from build123d import *

# Parameters (mm, degrees)
SKETCH1_R           = 278.5
BOSS_EXTRUDE1_DEPTH = 2.25
FILLET1_R           = 13


with BuildPart() as part:
    # Sketch1 → Boss-Extrude1 (new body, symmetric)
    with BuildSketch(Plane.XY):
        Circle(SKETCH1_R)
        with BuildLine():
            Line((249.915485715, -6.5), (-249.915485715, -6.5))
            ThreePointArc((-249.915485715, -6.5), (0, -250), (249.915485715, -6.5))
        make_face(mode=Mode.SUBTRACT)
        with BuildLine():
            Line((249.915485715, 6.5), (-249.915485715, 6.5))
            ThreePointArc((-249.915485715, 6.5), (0, 250), (249.915485715, 6.5))
        make_face(mode=Mode.SUBTRACT)
    extrude(amount=BOSS_EXTRUDE1_DEPTH, both=True)

    # Fillet1
    fillet1_edges = [part.edges().sort_by_distance(p)[0] for p in [
        (-249.915485715, -6.5, 0),
        (249.915485715, -6.5, 0),
        (249.915485715, 6.5, 0),
        (-249.915485715, 6.5, 0),
    ]]
    fillet(fillet1_edges, radius=FILLET1_R)


solid = part.part
Design review of the part built by this model. Coordinates are the model's own, in mm. A direction names the side the tool comes from. Round coordinates to 2 decimals unless told otherwise and drop trailing zeros. Loops run counter-clockwise (first coordinate to the right, second up) from the corner with the lowest first, then second, coordinate; pieces in that order, holes last. Notation, with made-up numbers: (26.5, 62.25) - (38.5, 62.25) arc R30 ccw to (38.5, 101.25) - close; hole circle Ø9 at (76.25, -15.5). An arc over 180 degrees is marked (long way). One line per question, with ' | ' between items.
1. Clearance check with flat-ended pins moving along their axes: P1, Ø2, axis at x = 133, z = -0.5, coming from the +Y side; P2, Ø1.5, axis at x = 150, z = -1.5, coming from the +Y side; P3, Ø1, axis at y = 180, z = 0, coming from the -X side. State where each tip first meets the part, or that it passes through.
Results are:
P1: stops at y = 245.23 | P2: stops at y = 235.13 | P3: stops at x = -212.94
2. We need section D-D, the plane x = 199. State the section outline as (y, z) points, and give its area (3 significant figures).
Results are:
outline: (-194.84, -2.25) - (-151.32, -2.25) - (-151.32, 2.25) - (-194.84, 2.25) - close; (-6.5, -2.25) - (6.5, -2.25) - (6.5, 2.25) - (-6.5, 2.25) - close; (151.32, -2.25) - (194.84, -2.25) - (194.84, 2.25) - (151.32, 2.25) - close | area: 450 mm²
3. We need section C-C, the plane z = 0.2. State the section outline as (x, y) points.
Results are:
outline: circle Ø557 at (0, 0); hole (-249.15, -20.57) arc R250 ccw to (249.15, -20.57) arc R13 ccw to (236.2, -6.5) - (-236.2, -6.5) arc R13 ccw to start; hole (-249.15, 20.57) arc R13 ccw to (-236.2, 6.5) - (236.2, 6.5) arc R13 ccw to (249.15, 20.57) arc R250 ccw to start
4. We need section A-A, the plane x = 0. State the section outline as (y, z) points, and give its area (3 significant figures).
Results are:
outline: (-278.5, -2.25) - (-250, -2.25) - (-250, 2.25) - (-278.5, 2.25) - close; (-6.5, -2.25) - (6.5, -2.25) - (6.5, 2.25) - (-6.5, 2.25) - close; (250, -2.25) - (278.5, -2.25) - (278.5, 2.25) - (250, 2.25) - close | area: 315 mm²
5. For faces 4 (the face through (-245.861, -10.805, -0.031)), 5 (the face through (-43, 1, 2.25)), list the 3-axis set-ups (+Z, -Z, +X, -X, +Y, -Y) from which the entire face can be reached by the end or side of a thin tool; tool diameter is ignored.
Results are:
face 4: +Z, -Z | face 5: +Z, +X, -X, +Y, -Y
6. Draft analysis for pull direction Y (two halves, no side actions). For faces 1 (the face through (-221.01, -169.46, 0.03)), 2 (the face through (-43, 1, -2.25)), 3 (the face through (-245.657, 10.584, -0.031)), state which applies: released by +Y, released by -Y, zero draft, split by the parting line, or undercut.
Results are:
face 1: split by the parting line | face 2: zero draft | face 3: undercut
7. For L1, parallel to Y at x = 2, z = -1.85; L2, parallel to Y at x = 224, z = -1; L3, parallel to X at y = -115, z = 2.1, list the stretches that pass through material, from the lowest coordinate up. Write a range as [from, to].
Results are:
L1: y = [-278.49, -249.99], [-6.5, 6.5], [249.99, 278.49] | L2: y = [-165.49, -111.01], [-6.5, 6.5], [111.01, 165.49] | L3: x = [-253.65, -221.98], [221.98, 253.65]
8. We need section B-B, the plane y = 137. State the section outline as (x, z) points.
Results are:
outline: (-242.47, -2.25) - (-209.12, -2.25) - (-209.12, 2.25) - (-242.47, 2.25) - close; (209.12, -2.25) - (242.47, -2.25) - (242.47, 2.25) - (209.12, 2.25) - close
